Can you work these out from the model? Positions are in its coordinate system, mm. Give positions to 0.01 mm unless a question says otherwise; leave off trailing zeros. Write each loop counter-clockwise with the first axis right and the second up, starting at its lowest first coordinate (ties: lowest second). Pieces come first, ordered by that corner, then holes. Notation, with made-up numbers: M 54.5,64.25 L 81.5,64.25 A12 cw 81.5,77.25 Z; hole C -12,-24.75 d7. An arc over 180 degrees is marked long. Write each question's results on one line, items separated by ' | '.
Solid Edge part; units mm, degrees
sketch "Sketch1" plane through (0, 0, 0) normal (0, 0, 1) x (1, 0, 0)
  line L0 (-304.8, -609.6) -> (304.8, -609.6)
  line L1 (304.8, -609.6) -> (304.8, 0)
  line L2 (304.8, 0) -> (-304.8, 0)
  line L3 (-304.8, 0) -> (-304.8, -609.6)
  dimension "D1" = 304.8
  dimension "D2" = 304.8
extrude "Protrusion1" add sketch "Sketch1" along normal blind 6.35
extrude "Cutout1" [suppressed]
sketch "Sketch2" plane through (0, -304.8, 6.35) normal (0, 0, 1) x (0, 1, 0)
  line L0 (212.725, -119.0625) -> (-304.8, -119.0625)
  line L1 (-304.8, -119.0625) -> (-304.8, 119.0625)
  line L2 (-304.8, 119.0625) -> (212.725, 119.0625)
  line L3 (212.725, 119.0625) -> (212.725, -119.0625)
  dimension "D1" = 304.8
  dimension "D2" = 304.8
extrude "Cutout2" cut sketch "Sketch2" against normal through all
properties material "Wood, Pine"
Item 1: If I drill on line 1 (X direction, y = -452, z = 1.75); line 2 (Y direction, x = 39.5, z = 1) (3 decimals), over which ranges is the centre line in solid material (lowest first)? Write a range as from..to.
Geometry says:
line 1: x = -304.8..-119.06, 119.06..304.8 | line 2: y = -92.075..0
Item 2: I want a section at B-B, the plane z = 2.5. Please give me the cut outline in (x, y) (1 decimal).
Geometry says:
outline: M -304.8,-609.6 L -119.1,-609.6 L -119.1,-92.1 L 119.1,-92.1 L 119.1,-609.6 L 304.8,-609.6 L 304.8,0 L -304.8,0 Z
Item 3: I'm going to push a flat-ended pin straight in: pin 1 (1 mm diameter, centred on x = -110, z = 4.5, fed in from -Y) (3 decimals). Where does the tip first touch, or does it pass through?
Geometry says:
pin 1: stops at y = -92.075
Item 4: I want a section at C-C, the plane x = -5. Please give me the cut outline in (y, z) (3 decimals).
Geometry says:
outline: M -92.075,0 L 0,0 L 0,6.35 L -92.075,6.35 Z
Item 5: I want a section at A-A, the plane y = -468.5. Please give me the cut outline in (x, z).
Geometry says:
outline: M -304.8,0 L -119.06,0 L -119.06,6.35 L -304.8,6.35 Z; M 119.06,0 L 304.8,0 L 304.8,6.35 L 119.06,6.35 Z
